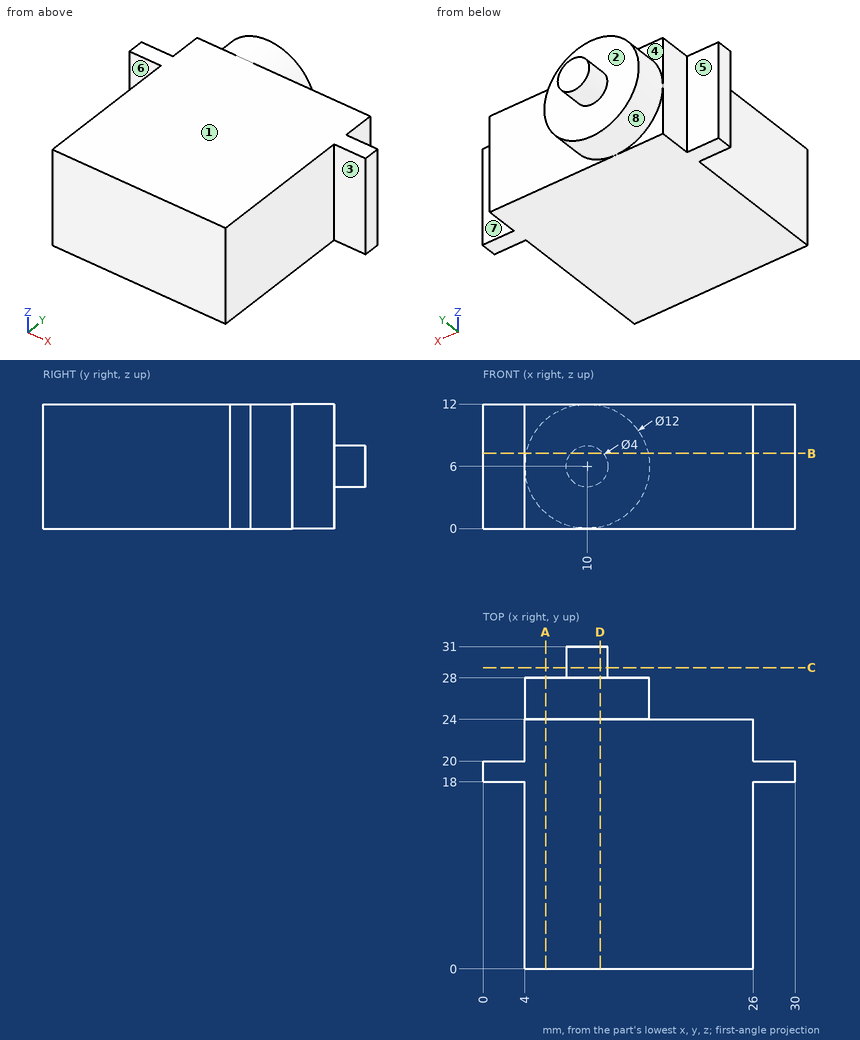
Print and shaded views of the part. All mm, measured from the part's lowest x, y and z. A direction names the side the tool comes from. Coordinates: 2 decimals unless noted, no trailing zeros. Write each loop counter-clockwise with the first axis right and the second up, starting at its lowest first coordinate (ties: lowest second). Pieces come first, ordered by that corner, then holes.
(1) Drill centre lines: probe 1 along X at (y, z) = (23, 0.5); probe 2 along Y at (x, z) = (11.5, 1.5); probe 3 along Y at (x, z) = (17.75, 3). Where is each one in solid material? Low to high.
(2) Flat gauge pins, fed straight in: pin 1 (1.2 mm diameter, centred on y = 22, z = 4, fed in from -X); pin 2 (6 mm diameter, centred on y = 12, z = 5, fed in from +X); pin 3 (3 mm diameter, centred on x = 1.5, z = 5, fed in from +Y). Where does each tip first touch, or does it go through?
(3) Cut at C-C, the plane y = 29. List the corners of the cut face in (x, z), and give its area (3 significant figures).
(4) 3-axis set-ups, long thin cutter, end or side, ignore diameter. For the marked faces 4, 5, 6, 7 and 8: which of +Z, -Z, +X, -X, +Y, -Y reach the whole face in a straight line?
(5) Cut at A-A, the plane x = 6. List the corners of the cut face in (y, z).
(6) Cut at D-D, the plane x = 11.25. List the corners of the cut face in (y, z).
(7) Cut at B-B, the plane z = 7.25. List the corners of the cut face in (x, y), and give its area (3 significant figures).
(8) Two-plate mould, pull along Y, no slides. Class the marked faces 1, 2 and 3: +Y half, -Y half, draft (parallel to the pull), parting line (faces both ways), or undercut.
Geometry says:
1. probe 1: x = 4 to 26
1. probe 2: y = 0 to 28
1. probe 3: y = 0 to 24
2. pin 1: stops at x = 4
2. pin 2: stops at x = 26
2. pin 3: stops at y = 20
3. outline: circle Ø4 at (10, 6)
3. area: 12.6 mm2
4. face 4: +Z, -X, +Y
4. face 5: +Z, -Z, -X, +Y
4. face 6: +Z, -Z, -X, -Y
4. face 7: +Z, -Z, +X, +Y
4. face 8: +Y
5. outline: (0, 0) - (24, 0) - (24, 1.53) - (28, 1.53) - (28, 10.47) - (24, 10.47) - (24, 12) - (0, 12) - close
6. outline: (0, 0) - (24, 0) - (24, 0.13) - (28, 0.13) - (28, 4.44) - (31, 4.44) - (31, 7.56) - (28, 7.56) - (28, 11.87) - (24, 11.87) - (24, 12) - (0, 12) - close
7. outline: (0, 18) - (4, 18) - (4, 0) - (26, 0) - (26, 18) - (30, 18) - (30, 20) - (26, 20) - (26, 24) - (15.87, 24) - (15.87, 28) - (11.56, 28) - (11.56, 31) - (8.44, 31) - (8.44, 28) - (4.13, 28) - (4.13, 24) - (4, 24) - (4, 20) - (0, 20) - close
7. area: 600 mm2
8. face 1: draft
8. face 2: +Y half
8. face 3: -Y half
